```python
from build123d import *

# Parameters (mm, degrees)
BOSS_EXTRUDE1_DEPTH                 = 200
F_3_32_0_09375_DIAMETER_HOLE1_D     = 2.38125
F_3_32_0_09375_DIAMETER_HOLE1_DEPTH = 5
F_3_32_0_09375_DIAMETER_HOLE1_TIP   = 0.715399675
F_3_32_0_09375_DIAMETER_HOLE2_D     = 2.38125
F_3_32_0_09375_DIAMETER_HOLE2_DEPTH = 5
F_3_32_0_09375_DIAMETER_HOLE2_TIP   = 0.715399675


with BuildPart() as part:
    # Sketch1 → Boss-Extrude1 (new body)
    with BuildSketch(Plane.XY):
        Polygon((-6.38902439, -3.969512195), (5.31097561, -3.969512195), (5.31097561, 7.730487805), (6.31097561, 7.730487805), (6.31097561, -4.969512195), (-6.38902439, -4.969512195), align=None)
    extrude(amount=BOSS_EXTRUDE1_DEPTH)

    # 3/32 (0.09375) Diameter Hole1
    with Locations(Plane(origin=(0, -3.969512195, 0), x_dir=(1, 0, 0), z_dir=(0, 1, 0))):
        with Locations((-0.53902439, -4.970860359), (-0.53902439, -100), (-0.53902439, -195)):
            Hole(F_3_32_0_09375_DIAMETER_HOLE1_D / 2, depth=F_3_32_0_09375_DIAMETER_HOLE1_DEPTH)
            with Locations((0, 0, -(F_3_32_0_09375_DIAMETER_HOLE1_DEPTH + F_3_32_0_09375_DIAMETER_HOLE1_TIP / 2))):  # 118° drill point
                Cone(0, F_3_32_0_09375_DIAMETER_HOLE1_D / 2, F_3_32_0_09375_DIAMETER_HOLE1_TIP, mode=Mode.SUBTRACT)

    # 3/32 (0.09375) Diameter Hole2
    with Locations(Plane.ZY.offset(-5.31097561)):
        with Locations((65, 1.880487805), (135, 1.880487805)):
            Hole(F_3_32_0_09375_DIAMETER_HOLE2_D / 2, depth=F_3_32_0_09375_DIAMETER_HOLE2_DEPTH)
            with Locations((0, 0, -(F_3_32_0_09375_DIAMETER_HOLE2_DEPTH + F_3_32_0_09375_DIAMETER_HOLE2_TIP / 2))):  # 118° drill point
                Cone(0, F_3_32_0_09375_DIAMETER_HOLE2_D / 2, F_3_32_0_09375_DIAMETER_HOLE2_TIP, mode=Mode.SUBTRACT)


solid = part.part
```
Input: part model. Units: mm. Frame: model coordinates. A direction names the side the tool comes from. Give positions to 0.01 mm unless a question says otherwise; leave off trailing zeros. Order: outer loops, then holes, each group sorted by start corner. A loop starts at its lowest first (then second) coordinate and runs counter-clockwise, first axis right, second up.
1. Cut plane B-B (x = -3.75). Return loops of the section in (y, z), and give its area (3 significant figures).
Computed:
outline: (-4.97, 0) - (-3.97, 0) - (-3.97, 200) - (-4.97, 200) - close
area: 200 mm2
2. Pin query (flat end, axial travel): pin 1 Ø4 at (x, z) = (-0.5, 112.5) entering from +Y; pin 2 Ø4 at (y, z) = (1.88, 135) entering from -X. Return the tip coordinate at first contact, or that it passes through.
Computed:
pin 1: stops at y = -3.97
pin 2: stops at x = 5.31
3. Set-up query: faces 1 (the face through (5.311, 2, 99)), 2 (the face through (6, -1, 0)). Return all of +Z, -Z, +X, -X, +Y, -Y with unobstructed straight access to the full face (end or side cutting, diameter ignored); none if empty.
Computed:
face 1: +Z, -Z, -X, +Y
face 2: -Z, +X, -X, +Y, -Y
4. Line query: probe 1 along X at (y, z) = (-4.65, 100); probe 2 along Y at (x, z) = (5.7, 65); probe 3 along X at (y, z) = (-1.75, 25.5). Output: solid intervals per line, ascending.
Computed:
probe 1: x = -6.39 to -1.73, 0.65 to 6.31
probe 2: y = -4.97 to 0.69, 3.07 to 7.73
probe 3: x = 5.31 to 6.31
5. Cut plane A-A (z = 180.5). Return loops of the section in (x, y).
Computed:
outline: (-6.39, -4.97) - (6.31, -4.97) - (6.31, 7.73) - (5.31, 7.73) - (5.31, -3.97) - (-6.39, -3.97) - close
